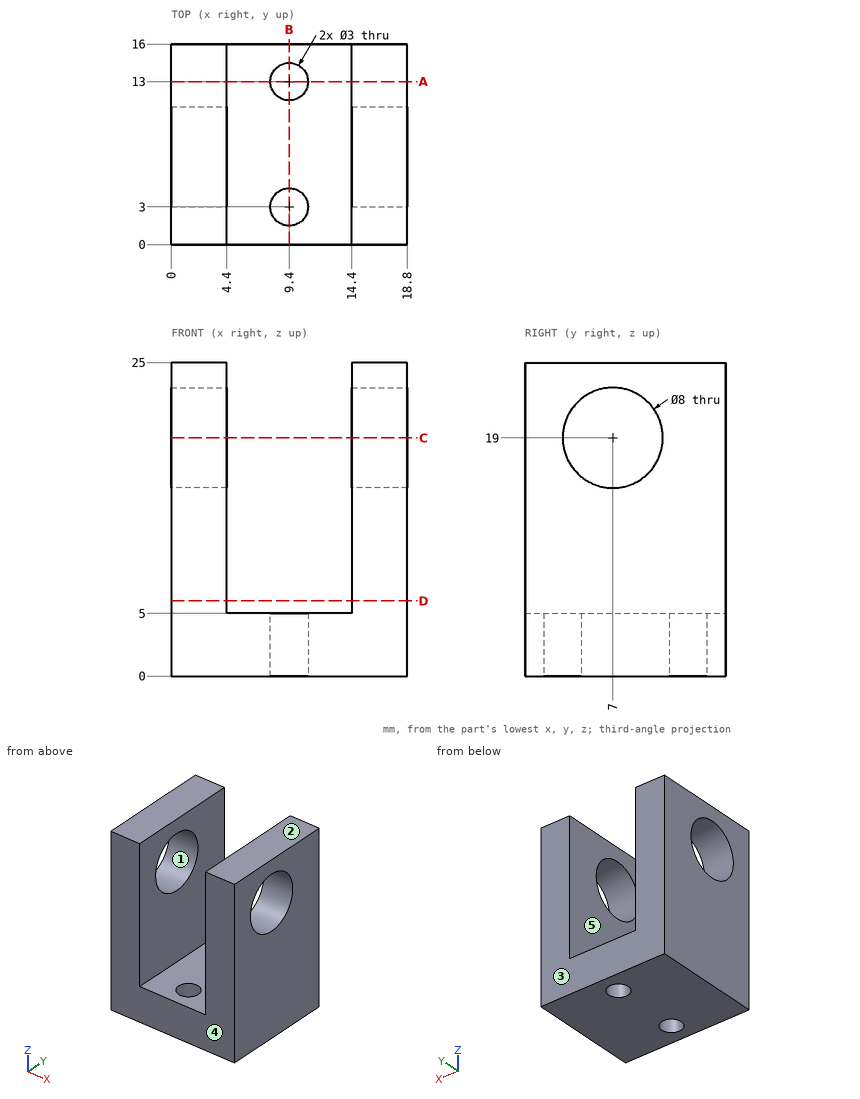
Print and shaded views of the part. All mm, measured from the part's lowest x, y and z. A direction names the side the tool comes from. Give positions to 0.01 mm unless a question says otherwise; leave off trailing zeros. Loops run counter-clockwise (first coordinate to the right, second up) from the corner with the lowest first, then second, coordinate; pieces in that order, holes last. Notation, with made-up numbers: (18, 74) - (38, 74) arc R33 cw to (38, 106) - close; hole circle Ø2 at (22.5, 62.25). An arc over 180 degrees is marked (long way). One line per item, written item: value. Start each with the question number.
1. Pin check, flat tips, straight feed: pin 1 (5 mm diameter, centred on x = 8, y = 4.5, fed in from +Z); pin 2 (4 mm diameter, centred on x = 14, z = 12, fed in from -Y). Stop position of each tip, or through.
2. Slice it at B-B (x = 9.4). List the corners of the cut face in (y, z), plus the area to 3 significant figures.
3. Probe L1, parallel to Y at x = 9.4, z = 3.3; L2, parallel to X at y = 3.25, z = 15.75; L3, parallel to Y at x = 3.25, z = 19. List the from-to ranges inside material, lowest first. Write a range as from..to.
4. Slice it at D-D (z = 6). List the corners of the cut face in (x, y).
5. Pull direction Z, two halves, no side cores. Call the marked faces 1, 2 and 3: pulls with the +Z half, pulls with the -Z half, needs draft (parallel to the pull), parting line crosses it, or undercut.
6. Slice it at A-A (y = 13). List the corners of the cut face in (x, z).
7. Slice it at C-C (z = 19). List the corners of the cut face in (x, y), plus the area to 3 significant figures.
8. Which spindle directions (+Z, -Z, +X, -X, +Y, -Y) get a long thin tool onto all of the face, cutting with end or side? Do the marked faces 4 and 5. Say none if no direction does.
Solution:
1. pin 1: stops at z = 5
1. pin 2: stops at y = 0
2. outline: (0, 0) - (1.5, 0) - (1.5, 5) - (0, 5) - close; (4.5, 0) - (11.5, 0) - (11.5, 5) - (4.5, 5) - close; (14.5, 0) - (16, 0) - (16, 5) - (14.5, 5) - close
2. area: 50.0 mm^2
3. L1: y = 0..1.5, 4.5..11.5, 14.5..16
3. L2: x = 0..4.4, 14.4..18.8
3. L3: y = 0..3, 11..16
4. outline: (0, 0) - (4.4, 0) - (4.4, 16) - (0, 16) - close; (14.4, 0) - (18.8, 0) - (18.8, 16) - (14.4, 16) - close
5. face 1: undercut
5. face 2: pulls with the +Z half
5. face 3: needs draft
6. outline: (0, 0) - (7.9, 0) - (7.9, 5) - (4.4, 5) - (4.4, 25) - (0, 25) - close; (10.9, 0) - (18.8, 0) - (18.8, 25) - (14.4, 25) - (14.4, 5) - (10.9, 5) - close
7. outline: (0, 0) - (4.4, 0) - (4.4, 3) - (0, 3) - close; (0, 11) - (4.4, 11) - (4.4, 16) - (0, 16) - close; (14.4, 0) - (18.8, 0) - (18.8, 3) - (14.4, 3) - close; (14.4, 11) - (18.8, 11) - (18.8, 16) - (14.4, 16) - close
7. area: 70.4 mm^2
8. face 4: +Z, -Z, +X, -X, -Y
8. face 5: +Z, +Y, -Y
